Part model, mm, in its own coordinate system. Round coordinates to 2 decimals unless told otherwise and drop trailing zeros. Write each loop counter-clockwise with the first axis right and the second up, starting at its lowest first coordinate (ties: lowest second). Pieces come first, ordered by that corner, then holes. Notation, with made-up numbers: M -8.75,-4.5 L 43.25,-4.5 A28 cw 43.25,17.5 Z; hole C 3.25,54.25 d2. An arc over 180 degrees is marked long. One line per question, with ' | ' between items. Start each with the question number.
1) Saw through at A-A (x = 6.25). List the corners of the cut face in (y, z), plus the area to 3 significant figures.
2) Drop flat-ended pins along their axis: pin 1 Ø0.8 at (x, y) = (0.5, 1) entering from -Z; pin 2 Ø1 at (y, z) = (1.5, -36) entering from +X. Give the stop position or say it passes through.
3) Saw through at C-C (y = 1.55). List the corners of the cut face in (x, z).
4) Wall check: probe 1 along Z at (x, y) = (12.25, 0.25); probe 2 along Z at (x, y) = (4.5, 0.3); probe 3 along X at (y, z) = (1.9, -34). Give the ranges that are in metal, low to high. Write a range as [from, to].
5) Saw through at B-B (z = -17.5). List the corners of the cut face in (x, y), plus the area to 3 significant figures.
6) Saw through at D-D (x = 15.25). List the corners of the cut face in (y, z), plus the area to 3 significant figures.
```python
from build123d import *

# Parameters (mm, degrees)
SKETCH_1_W      = 7.6
SKETCH_1_H      = 2.1
EXTRUDE_1_DEPTH = 2


with BuildPart() as part:
    # 草图1 → 凸台-拉伸1 (new body)
    with BuildSketch(Plane(origin=(0, 0, 0), x_dir=(1, 0, 0), z_dir=(0, 1, 0))):
        Polygon((0, 33.8), (0, 0), (5, 0), (5, -2), (12.6, -2), (12.6, 0), (17.6, 0), (17.6, 34.8), (12.6, 34.8), (12.6, 36.8), (5, 36.8), (5, 34.8), (1, 34.8), (1, 33.8), align=None)
        with Locations((8.8, 17.95)):
            Rectangle(SKETCH_1_W, SKETCH_1_H, mode=Mode.SUBTRACT)
    extrude(amount=EXTRUDE_1_DEPTH)


solid = part.part
```
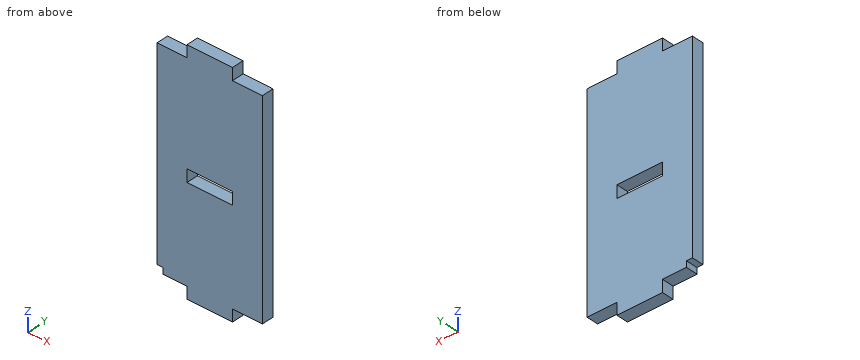
Answer key:
1) outline: M 0,-36.8 L 2,-36.8 L 2,-19 L 0,-19 Z; M 0,-16.9 L 2,-16.9 L 2,2 L 0,2 Z | area: 73.4 mm2
2) pin 1: stops at z = -33.8 | pin 2: stops at x = 12.6
3) outline: M 0,-33.8 L 1,-33.8 L 1,-34.8 L 5,-34.8 L 5,-36.8 L 12.6,-36.8 L 12.6,-34.8 L 17.6,-34.8 L 17.6,0 L 12.6,0 L 12.6,2 L 5,2 L 5,0 L 0,0 Z; hole M 5,-19 L 12.6,-19 L 12.6,-16.9 L 5,-16.9 Z
4) probe 1: z = [-36.8, -19], [-16.9, 2] | probe 2: z = [-34.8, 0] | probe 3: x = [1, 17.6]
5) outline: M 0,0 L 5,0 L 5,2 L 0,2 Z; M 12.6,0 L 17.6,0 L 17.6,2 L 12.6,2 Z | area: 20.0 mm2
6) outline: M 0,-34.8 L 2,-34.8 L 2,0 L 0,0 Z | area: 69.6 mm2
